from build123d import *

# Parameters (mm, degrees)
EXTRUDE_1_DEPTH     = 40
SKETCH_2_W          = 25
SKETCH_2_H          = 47
EXTRUDE_2_DEPTH     = 40
HOLE_WIZARD_3_D     = 23
EXTRUDE_3_DEPTH     = 40
EXTRUDE_5_DEPTH     = 20
HOLE_WIZARD_4_D     = 5.2
SKETCH_15_R         = 3
CUT_EXTRUDE_1_DEPTH = 3


with BuildPart() as part:
    # 草图1 → 凸台-拉伸1 (new body)
    with BuildSketch(Plane.XY):
        Polygon((13.1, -5.375), (13.1, -25.375), (10.1, -25.375), (10.1, -5.375), (-10.1, -5.375), (-10.1, -25.375), (-13.1, -25.375), (-13.1, -5.375), (-25, -5.375), (-25, 5.375), (25, 5.375), (25, -5.375), align=None)
    extrude(amount=EXTRUDE_1_DEPTH)

    # 草图2 → 凸台-拉伸2 (add)
    with BuildSketch(Plane(origin=(0, 0, 0), x_dir=(-1, 0, 0), z_dir=(0, 0, -1))):
        with Locations((0, 28.875)):
            Rectangle(SKETCH_2_W, SKETCH_2_H)
    extrude(amount=-EXTRUDE_2_DEPTH)

    # 孔3 (through all)
    with Locations(Plane.XY.offset(40)):
        with Locations((0, 35.625)):
            Hole(HOLE_WIZARD_3_D / 2)

    # 草图10 → 凸台-拉伸3 (add)
    with BuildSketch(Plane.XY.offset(40)):
        Polygon((12.5, 35.375), (17.5, 35.375), (25, 15.375), (25, 5.375), (12.5, 5.375), align=None)
        Polygon((-12.5, 35.375), (-12.5, 5.375), (-25, 5.375), (-25, 15.375), (-17.5, 35.375), align=None)
    extrude(amount=-EXTRUDE_3_DEPTH)

    # 草图12 → 凸台-拉伸5 (add)
    with BuildSketch(Plane.XY.offset(40)):
        Polygon((12.5, 52.375), (17.5, 35.375), (12.5, 35.375), align=None)
        Polygon((-12.5, 52.375), (-17.5, 35.375), (-12.5, 35.375), align=None)
    extrude(amount=-EXTRUDE_5_DEPTH)

    # 孔4 (through all)
    with Locations(Plane(origin=(13.1, 0, 0), x_dir=(0, 0, -1), z_dir=(1, 0, 0))):
        with Locations((-31, -15.375), (-9, -15.375)):
            Hole(HOLE_WIZARD_4_D / 2)

    # 草图15 → 切除-拉伸1 (cut)
    with BuildSketch(Plane.XY.offset(40)):
        with Locations((-15.5, 51.125)):
            Circle(SKETCH_15_R)
        with Locations((15.5, 51.125)):
            Circle(SKETCH_15_R)
        with Locations((-15.5, 20.125)):
            Circle(SKETCH_15_R)
        with Locations((15.5, 20.125)):
            Circle(SKETCH_15_R)
    extrude(amount=-CUT_EXTRUDE_1_DEPTH, mode=Mode.SUBTRACT)


solid = part.part
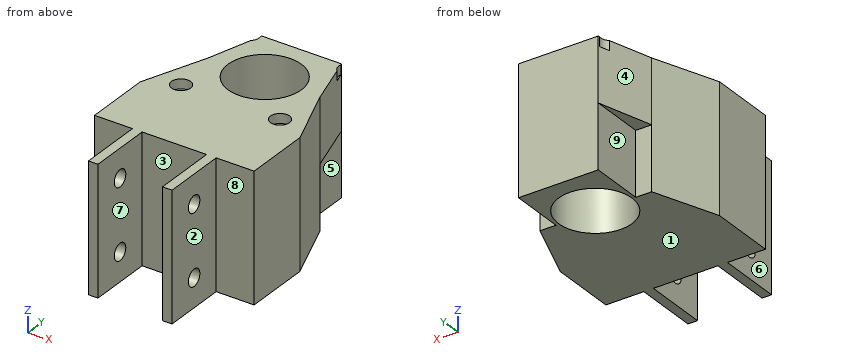
CAD build for the part. Positions are in the model's coordinates, mm. Face numbers are marked on the shaded views. A direction names the side the tool comes from. Coordinates: 2 decimals unless noted, no trailing zeros. Order: outer loops, then holes, each group sorted by start corner. A loop starts at its lowest first (then second) coordinate and runs counter-clockwise, first axis right, second up. Notation, with made-up numbers: (-0.5, 4) -> (12.5, 4) arc R21 ccw to (12.5, 9) -> close; hole circle Ø10 at (46.5, 64.25). An arc over 180 degrees is marked (long way). Answer in a Markdown table with one row per item.
1) Which spindle directions (+Z, -Z, +X, -X, +Y, -Y) get a long thin tool onto all of the face, cutting with end or side? Do the marked faces 5, 6, 7, 8 and 9. Say none if no direction does.
Check values:
| item | result |
|---|---|
| face 5 | -Z, +X, +Y |
| face 6 | +Z, -Z, -X, -Y |
| face 7 | +Z, -Z, -Y |
| face 8 | +Z, -Z, +X, -Y |
| face 9 | -Z, -X, +Y |
2) Band-saw the part on A-A (x = 0). List the corners of the cut face in (y, z) (3 decimals), and give its area (3 significant figures).
Check values:
| item | result |
|---|---|
| outline | (-5.375, 0) -> (24.125, 0) -> (24.125, 40) -> (-5.375, 40) -> close; (47.125, 0) -> (52.375, 0) -> (52.375, 40) -> (47.125, 40) -> close |
| area | 1,390 mm2 |
3) Flat gauge pins, fed straight in: P1, Ø5, axis at x = 17.5, z = 5.5, coming from the +Y side (3 decimals); P2, Ø9.5, axis at x = -15.5, y = 20.125, coming from the -Z side; P3, Ø4, axis at y = 40.5, z = 27, coming from the +X side; P4, Ø9.5, axis at x = 19.5, z = 24.5, coming from the -Y side (3 decimals). Where does each tip first touch, or does it go through?
Check values:
| item | result |
|---|---|
| P1 | y = 35.375 |
| P2 | z = 0 |
| P3 | x = 16.58 |
| P4 | y = -5.375 |
4) Band-saw the part on C-C (y = -8.5). List the corners of the cut face in (x, z), and give its area (3 significant figures).
Check values:
| item | result |
|---|---|
| outline | (-13.1, 0) -> (-10.1, 0) -> (-10.1, 40) -> (-13.1, 40) -> close; (10.1, 0) -> (13.1, 0) -> (13.1, 40) -> (10.1, 40) -> close |
| area | 240 mm2 |
5) Drill centre lines: line 1 (Y direction, x = 0, z = 21.5) (3 decimals); line 2 (Z direction, x = -13.5, y = 38); line 3 (Y direction, x = 15, z = 2.5) (3 decimals). Where is each one in solid material? Low to high.
Check values:
| item | result |
|---|---|
| line 1 | -5.375 to 24.125, 47.125 to 52.375 |
| line 2 | 20 to 40 |
| line 3 | -5.375 to 35.375 |
6) Band-saw the part on B-B (z = 31). List the corners of the cut face in (x, y) (3 decimals).
Check values:
| item | result |
|---|---|
| outline | (-25, -5.375) -> (-13.1, -5.375) -> (-13.1, -12.775) -> (-10.1, -12.775) -> (-10.1, -5.375) -> (10.1, -5.375) -> (10.1, -12.775) -> (13.1, -12.775) -> (13.1, -5.375) -> (25, -5.375) -> (25, 15.375) -> (17.5, 35.375) -> (12.5, 52.375) -> (-12.5, 52.375) -> (-17.5, 35.375) -> (-25, 15.375) -> close; (-13.1, -25.375) -> (-10.1, -25.375) -> (-10.1, -17.975) -> (-13.1, -17.975) -> close; (10.1, -25.375) -> (13.1, -25.375) -> (13.1, -17.975) -> (10.1, -17.975) -> close; hole circle Ø23 at (0, 35.625) |
7) Mould opens along X. For the marked faces 1, 2, 3 and 4 say: pulls with the +X half, pulls with the -X half, needs draft (parallel to the pull), parting line crosses it, or undercut.
Check values:
| item | result |
|---|---|
| face 1 | needs draft |
| face 2 | pulls with the +X half |
| face 3 | undercut |
| face 4 | pulls with the -X half |
8) Band-saw the part on D-D (z = 16). List the corners of the cut face in (x, y) (3 decimals), and give its area (3 significant figures).
Check values:
| item | result |
|---|---|
| outline | (-25, -5.375) -> (-13.1, -5.375) -> (-13.1, -25.375) -> (-10.1, -25.375) -> (-10.1, -5.375) -> (10.1, -5.375) -> (10.1, -25.375) -> (13.1, -25.375) -> (13.1, -5.375) -> (25, -5.375) -> (25, 15.375) -> (17.5, 35.375) -> (12.5, 35.375) -> (12.5, 52.375) -> (-12.5, 52.375) -> (-12.5, 35.375) -> (-17.5, 35.375) -> (-25, 15.375) -> close; hole circle Ø23 at (0, 35.625) |
| area | 2,020 mm2 |
